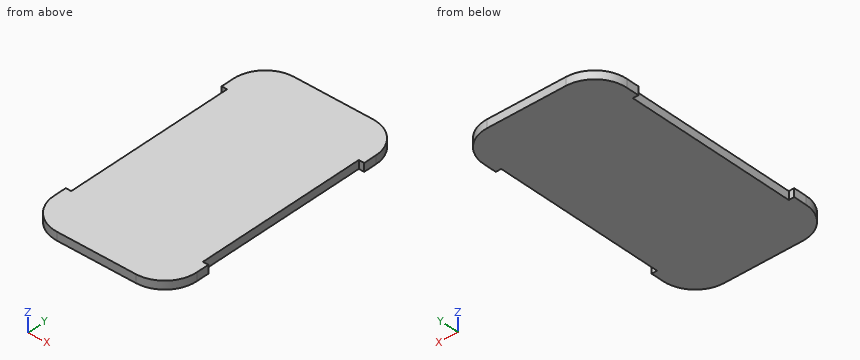
from build123d import *

# Parameters (mm, degrees)
EXTRUDE1_DEPTH = 0.9


with BuildPart() as part:
    # Sketch1 → Extrude1 (new body)
    with BuildSketch(Plane(origin=(0, 0, 4.2), x_dir=(-1, 0, 0), z_dir=(0, 0, -1))):
        with BuildLine():
            Line((-55.7, 309.3), (-64.3, 309.3))
            ThreePointArc((-64.3, 309.3), (-66.774873734, 308.274873734), (-67.8, 305.8))
            Line((-67.8, 305.8), (-67.8, 304.4))
            Line((-67.8, 304.4), (-67.2, 304.4))
            Line((-67.2, 304.4), (-67.2, 285.6))
            Line((-67.2, 285.6), (-67.8, 285.6))
            Line((-67.8, 285.6), (-67.8, 284.2))
            ThreePointArc((-67.8, 284.2), (-66.774873734, 281.725126266), (-64.3, 280.7))
            Line((-64.3, 280.7), (-55.7, 280.7))
            ThreePointArc((-55.7, 280.7), (-53.225126266, 281.725126266), (-52.2, 284.2))
            Line((-52.2, 284.2), (-52.2, 285.6))
            Line((-52.2, 285.6), (-52.8, 285.6))
            Line((-52.8, 285.6), (-52.8, 304.4))
            Line((-52.8, 304.4), (-52.2, 304.4))
            Line((-52.2, 304.4), (-52.2, 305.8))
            ThreePointArc((-52.2, 305.8), (-53.225126266, 308.274873734), (-55.7, 309.3))
        make_face()
    extrude(amount=-EXTRUDE1_DEPTH)


solid = part.part
For this review, take the finished solid that the model builds, in its own axes (mm). Give positions to 0.01 mm unless a question says otherwise; leave off trailing zeros. Order: outer loops, then holes, each group sorted by start corner. A loop starts at its lowest first (then second) coordinate and runs counter-clockwise, first axis right, second up. Notation, with made-up numbers: (34.5, 69.5) -> (71.5, 69.5) arc R17 ccw to (71.5, 75.5) -> close; hole circle Ø2 at (-33.75, 76.5). An arc over 180 degrees is marked (long way). Write item = value, one per line.
1) We need section A-A, the plane z = 4.4. Give the boundary of the cut face in (x, y).
Findings:
outline = (52.2, 284.2) arc R3.5 ccw to (55.7, 280.7) -> (64.3, 280.7) arc R3.5 ccw to (67.8, 284.2) -> (67.8, 285.6) -> (67.2, 285.6) -> (67.2, 304.4) -> (67.8, 304.4) -> (67.8, 305.8) arc R3.5 ccw to (64.3, 309.3) -> (55.7, 309.3) arc R3.5 ccw to (52.2, 305.8) -> (52.2, 304.4) -> (52.8, 304.4) -> (52.8, 285.6) -> (52.2, 285.6) -> close
2) To check wall thickness, follow L1, parallel to X at y = 301.25, z = 4.3; L2, parallel to X at y = 306.75, z = 4.6; L3, parallel to Y at x = 54, z = 4.45. State the ranges of each line that lie inside material, in increasing order. Write a range as from..to.
Findings:
L1 = 52.8..67.2
L2 = 52.33..67.67
L3 = 281.14..308.86
3) Insertion check: pin 1 (0.5 mm diameter, centred on x = 52.5, z = 5, fed in from -Y). The pin has a flat end and moves straight along its axis. Give the tip position at first contact, or say it passes through.
Findings:
pin_1 = 282.32
4) We need section B-B, the plane y = 290. Give the boundary of the cut face in (x, z).
Findings:
outline = (52.8, 4.2) -> (67.2, 4.2) -> (67.2, 5.1) -> (52.8, 5.1) -> close
5) We need section C-C, the plane y = 283.25. Give the boundary of the cut face in (x, z), and give its area (3 significant figures).
Findings:
outline = (52.33, 4.2) -> (67.67, 4.2) -> (67.67, 5.1) -> (52.33, 5.1) -> close
area = 13.8 mm^2
